Source: CAD feature listing. Evaluate the final solid. Frame: model axes, mm. Coordinates: 2 decimals unless noted, no trailing zeros. Loops run counter-clockwise (first coordinate to the right, second up) from the corner with the lowest first, then second, coordinate; pieces in that order, holes last. Notation, with made-up numbers: (25, 87.25) - (44, 87.25) arc R23 cw to (44, 111.25) - close; hole circle Ø5 at (-26.75, 69). An arc over 180 degrees is marked (long way). Use one line per item in the form item = value. Start each with the question number.
from build123d import *

# Parameters (mm, degrees)
SKETCH1_W           = 3
SKETCH1_H           = 1
SKETCH1_W_2         = 1
SKETCH1_H_2         = 3
BOSS_EXTRUDE1_DEPTH = 30
SKETCH2_OUTSIDE_W   = 11.06
SKETCH2_OUTSIDE_H   = 11.06
SKETCH2_OUTSIDE_R   = 1.5
CUT_EXTRUDE1_DEPTH  = 30


with BuildPart() as part:
    # Sketch1 → Boss-Extrude1 (new body)
    with BuildSketch(Plane(origin=(0, 0, 0), x_dir=(1, 0, 0), z_dir=(0, 1, 0))):
        Rectangle(SKETCH1_W, SKETCH1_H)
        Rectangle(SKETCH1_W_2, SKETCH1_H_2)
    extrude(amount=BOSS_EXTRUDE1_DEPTH)

    # Sketch2 outside → Cut-Extrude1 (cut)
    with BuildSketch(Plane(origin=(0, 30, 0), x_dir=(1, 0, 0), z_dir=(0, 1, 0))):
        Rectangle(SKETCH2_OUTSIDE_W, SKETCH2_OUTSIDE_H)
        Circle(SKETCH2_OUTSIDE_R, mode=Mode.SUBTRACT)
    extrude(amount=-CUT_EXTRUDE1_DEPTH, mode=Mode.SUBTRACT)


solid = part.part
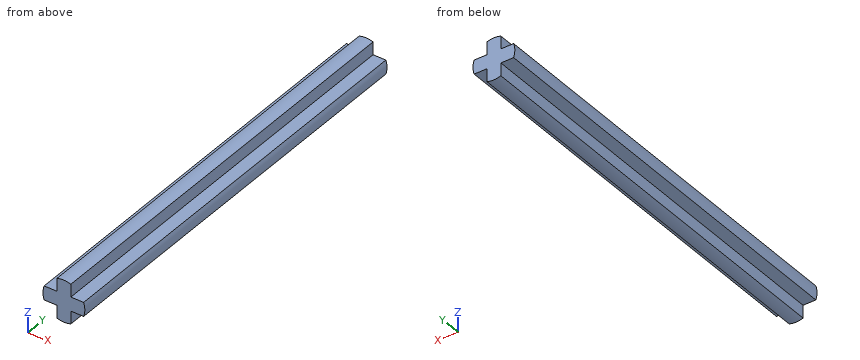
(1) Contact query for flat-ended pins moving along their axis: pin 1 (0.5 mm diameter, centred on x = -1, y = 10.5, fed in from +Z); pin 2 (0.5 mm diameter, centred on y = 20.5, z = -1, fed in from +X); pin 3 (0.7 mm diameter, centred on x = -1, y = 20, fed in from -Z). Output: stop coordinate, or through.
(2) Cut plane B-B, the plane z = -1. Output: boundary loops of the cut face in (x, y), plus the area to 3 significant figures.
(3) Cut plane A-A, the plane y = 3.25. Output: boundary loops of the cut face in (x, z), plus the area to 3 significant figures.
(4) Cut plane C-C, the plane x = 0.8. Output: boundary loops of the cut face in (y, z).
(5) Material intervals for line 1 (X direction, y = 18, z = -1.25); line 2 (X direction, y = 10.25, z = -0.1), sorted ascending.
Recorded:
q1.pin_1 = 0.5
q1.pin_2 = 0.5
q1.pin_3 = -0.5
q2.outline = (-0.5, 0) - (0.5, 0) - (0.5, 30) - (-0.5, 30) - close
q2.area = 30.0 mm²
q3.outline = (-1.41, -0.5) - (-0.5, -0.5) - (-0.5, -1.41) arc R1.5 ccw to (0.5, -1.41) - (0.5, -0.5) - (1.41, -0.5) arc R1.5 ccw to (1.41, 0.5) - (0.5, 0.5) - (0.5, 1.41) arc R1.5 ccw to (-0.5, 1.41) - (-0.5, 0.5) - (-1.41, 0.5) arc R1.5 ccw to start
q3.area = 4.89 mm²
q4.outline = (0, -0.5) - (30, -0.5) - (30, 0.5) - (0, 0.5) - close
q5.line_1 = -0.5 to 0.5
q5.line_2 = -1.5 to 1.5
